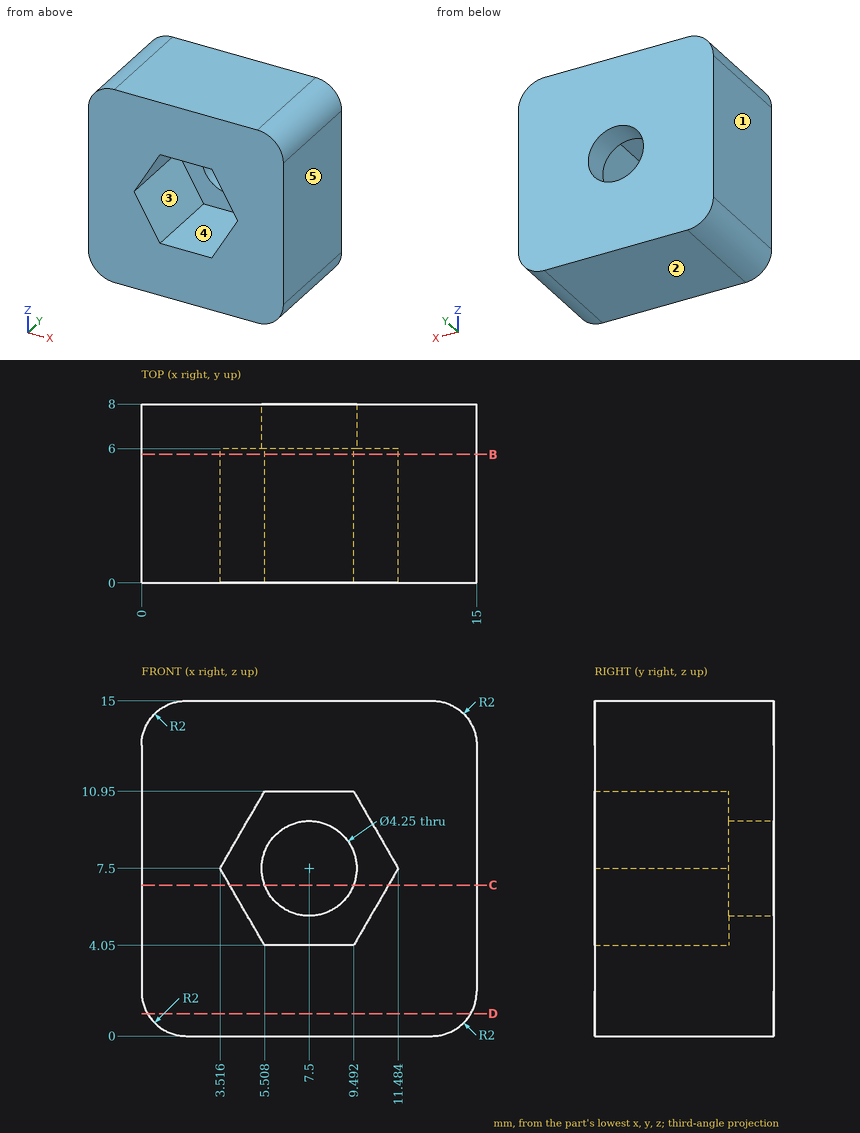
Study the drawing (mm; zero at the part's minimum x, y, z) and answer. A direction names the side the tool comes from. Give positions to 0.01 mm unless a question says otherwise; leave off trailing zeros. Loops run counter-clockwise (first coordinate to the right, second up) from the corner with the lowest first, then second, coordinate; pieces in that order, holes last. Notation, with made-up numbers: (35, -18) - (92, -18) arc R11 ccw to (92, -1) - close; hole circle Ø9 at (59, -37.75). An arc over 180 degrees is marked (long way). Answer in a Markdown table with one row per item. Add a question column.
Q1. This flat-tipped pin is pushed along its axis until it touches: P1, Ø2, axis at x = 8, z = 9, coming from the -Y side. Where does it stop, or does it pass through?
Q2. Consider line 1 along Z through (x, y) = (7.5, 7.4) (1 decimal); line 2 along Z through (x, y) = (9.25, 1). Determine where each line is inside the solid, lowest interval first.
Q3. The part is cut by section B-B (y = 5.75). Determine the outline of the cut face in (x, z), and give its area (3 significant figures).
Q4. The part is cut by section D-D (z = 1). Determine the outline of the cut face in (x, y), and give its area (3 significant figures).
Q5. A tool of negligible diameter and unlimited length cuts with its end or side. For the marked faces 4 and 5, from which of +Z, -Z, +X, -X, +Y, -Y can it reach the whole face along a straight path? Write none if from no direction.
Q6. Determine the mould class of the marked faces 1, 2 and 3 for opening direction X: released by +X, released by -X, zero draft, split by the parting line, or undercut.
Q7. The part is cut by section C-C (z = 6.75). Determine the outline of the cut face in (x, y).
Solution:
| question | item | result |
|---|---|---|
| 1 | P1 | stops at y = 6 |
| 2 | line 1 | z = 0 to 5.4, 9.6 to 15 |
| 2 | line 2 | z = 0 to 4.05, 10.95 to 15 |
| 3 | outline | (0, 2) arc R2 ccw to (2, 0) - (13, 0) arc R2 ccw to (15, 2) - (15, 13) arc R2 ccw to (13, 15) - (2, 15) arc R2 ccw to (0, 13) - close; hole (3.52, 7.5) - (5.51, 4.05) - (9.49, 4.05) - (11.48, 7.5) - (9.49, 10.95) - (5.51, 10.95) - close |
| 3 | area | 180 mm² |
| 4 | outline | (0.27, 0) - (14.73, 0) - (14.73, 8) - (0.27, 8) - close |
| 4 | area | 116 mm² |
| 5 | face 4 | -Y |
| 5 | face 5 | +Z, -Z, +X, +Y, -Y |
| 6 | face 1 | released by -X |
| 6 | face 2 | zero draft |
| 6 | face 3 | undercut |
| 7 | outline | (0, 0) - (3.95, 0) - (3.95, 6) - (5.51, 6) - (5.51, 8) - (0, 8) - close; (9.49, 6) - (11.05, 6) - (11.05, 0) - (15, 0) - (15, 8) - (9.49, 8) - close |
